from build123d import *

# Parameters (mm, degrees)
SKETCH1_W           = 22.84
SKETCH1_H           = 12.1
BOSS_EXTRUDE1_DEPTH = 17.2
BOSS_EXTRUDE2_DEPTH = 2.48
BOSS_EXTRUDE3_START = 2.48
SKETCH1_4_W         = 22.84
SKETCH1_4_H         = 12.1
BOSS_EXTRUDE3_DEPTH = 4.4
BOSS_EXTRUDE4_START = 6.88
SKETCH1_5_R         = 2.8
SKETCH1_5_R_2       = 6.05
SKETCH1_5_R_3       = 2.35
BOSS_EXTRUDE4_DEPTH = 4.28
BOSS_EXTRUDE5_START = 11.16
SKETCH1_6_R         = 2.35
BOSS_EXTRUDE5_DEPTH = 4.02


with BuildPart() as part:
    # Sketch1 → Boss-Extrude1 (new body)
    with BuildSketch(Plane(origin=(0, 0, 0), x_dir=(1, 0, 0), z_dir=(0, 1, 0))):
        with Locations((5.37, 0)):
            Rectangle(SKETCH1_W, SKETCH1_H)
    extrude(amount=-BOSS_EXTRUDE1_DEPTH)

    # Sketch1<3> → Boss-Extrude2 (add)
    with BuildSketch(Plane(origin=(0, 0, 0), x_dir=(1, 0, 0), z_dir=(0, 1, 0))):
        with BuildLine():
            Line((21.48, -6.05), (21.48, -1))
            Line((21.48, -1), (19.07, -1))
            ThreePointArc((19.07, -1), (18.07, 0), (19.07, 1))
            Line((19.07, 1), (21.48, 1))
            Line((21.48, 1), (21.48, 6.05))
            Line((21.48, 6.05), (-10.74, 6.05))
            Line((-10.74, 6.05), (-10.74, 1.33332999))
            Line((-10.74, 1.33332999), (-8.33, 1.33332999))
            ThreePointArc((-8.33, 1.33332999), (-6.99667001, 0), (-8.33, -1.33332999))
            Line((-8.33, -1.33332999), (-10.74, -1.33332999))
            Line((-10.74, -1.33332999), (-10.74, -6.05))
            Line((-10.74, -6.05), (21.48, -6.05))
        make_face()
    extrude(amount=BOSS_EXTRUDE2_DEPTH)

    # Sketch1<4> → Boss-Extrude3 (add)
    with BuildSketch(Plane(origin=(0, 0, 0), x_dir=(1, 0, 0), z_dir=(0, 1, 0)).offset(BOSS_EXTRUDE3_START)):
        with Locations((5.37, 0)):
            Rectangle(SKETCH1_4_W, SKETCH1_4_H)
    extrude(amount=BOSS_EXTRUDE3_DEPTH)

    # Sketch1<5> → Boss-Extrude4 (add)
    # profile 1 of 9: a face of its own
    with BuildSketch(Plane(origin=(0, 0, 0), x_dir=(1, 0, 0), z_dir=(0, 1, 0)).offset(BOSS_EXTRUDE4_START)):
        with Locations((7, 0)):
            Circle(SKETCH1_5_R)
    # profile 2 of 9: a face of its own
    with BuildSketch(Plane(origin=(0, 0, 0), x_dir=(1, 0, 0), z_dir=(0, 1, 0)).offset(BOSS_EXTRUDE4_START)):
        Circle(SKETCH1_5_R_2)
        Circle(SKETCH1_5_R_3, mode=Mode.SUBTRACT)
    # profile 3 of 9: a face of its own
    with BuildSketch(Plane(origin=(0, 0, 0), x_dir=(1, 0, 0), z_dir=(0, 1, 0)).offset(BOSS_EXTRUDE4_START)):
        with BuildLine():
            Line((4.691578101, -3.819894622), (7.957656401, -2.631139338))
            ThreePointArc((7.957656401, -2.631139338), (6.72964006, -2.786916845), (5.554464286, -2.398004691))
            ThreePointArc((5.554464286, -2.398004691), (5.172116481, -3.138743556), (4.691578101, -3.819894622))
        make_face()
    # profile 4 of 9: a face of its own
    with BuildSketch(Plane(origin=(0, 0, 0), x_dir=(1, 0, 0), z_dir=(0, 1, 0)).offset(BOSS_EXTRUDE4_START)):
        with BuildLine():
            ThreePointArc((5.554464286, 2.398004691), (6.72964006, 2.786916845), (7.957656401, 2.631139338))
            Line((7.957656401, 2.631139338), (4.691578101, 3.819894622))
            ThreePointArc((4.691578101, 3.819894622), (5.172116481, 3.138743556), (5.554464286, 2.398004691))
        make_face()
    # profile 5 of 9: a face of its own
    with BuildSketch(Plane(origin=(0, 0, 0), x_dir=(1, 0, 0), z_dir=(0, 1, 0)).offset(BOSS_EXTRUDE4_START)):
        Circle(SKETCH1_5_R_2)
    # profile 6 of 9: a face of its own
    with BuildSketch(Plane(origin=(0, 0, 0), x_dir=(1, 0, 0), z_dir=(0, 1, 0)).offset(BOSS_EXTRUDE4_START)):
        with Locations((7, 0)):
            Circle(SKETCH1_5_R)
    # profile 7 of 9: a face of its own
    with BuildSketch(Plane(origin=(0, 0, 0), x_dir=(1, 0, 0), z_dir=(0, 1, 0)).offset(BOSS_EXTRUDE4_START)):
        with Locations((7, 0)):
            Circle(SKETCH1_5_R)
    # profile 8 of 9: a face of its own
    with BuildSketch(Plane(origin=(0, 0, 0), x_dir=(1, 0, 0), z_dir=(0, 1, 0)).offset(BOSS_EXTRUDE4_START)):
        Circle(SKETCH1_5_R_2)
    # profile 9 of 9: a face of its own
    with BuildSketch(Plane(origin=(0, 0, 0), x_dir=(1, 0, 0), z_dir=(0, 1, 0)).offset(BOSS_EXTRUDE4_START)):
        Circle(SKETCH1_5_R_3)
    extrude(amount=BOSS_EXTRUDE4_DEPTH)

    # Sketch1<6> → Boss-Extrude5 (add)
    with BuildSketch(Plane(origin=(0, 0, 0), x_dir=(1, 0, 0), z_dir=(0, 1, 0)).offset(BOSS_EXTRUDE5_START)):
        with Locations(Location((0, 0, 0), (0, 0, 270))):
            Circle(SKETCH1_6_R)
    extrude(amount=BOSS_EXTRUDE5_DEPTH)


solid = part.part
Here's how the part is built. I have some questions about the finished solid (model axes, mm). A direction names the side the tool comes from. Round coordinates to 2 decimals unless told otherwise and drop trailing zeros. Loops run counter-clockwise (first coordinate to the right, second up) from the corner with the lowest first, then second, coordinate; pieces in that order, holes last.
1. We'd pull the mould along Z, two halves only. Please class faces 1 (the face through (-7.91, 2.48, -1.43)), 2 (the face through (-6.997, 1.223, -0.029)), 3 (the face through (6.347, 8.99, -3.217)), 4 (the face through (6.302, 8.99, 3.234)): +Z half, -Z half, draft (parallel to the pull), parting line (faces both ways), or undercut.
Answer list:
face 1: draft
face 2: undercut
face 3: -Z half
face 4: +Z half
2. If we section it at B-B on z = 0.5: Write out the boundary of the cut face in (x, y) (3 decimals).
Answer list:
outline: (-7.094, 0) - (-6.05, 0) - (-6.05, -17.2) - (16.79, -17.2) - (16.79, 0) - (18.204, 0) - (18.204, 2.48) - (16.79, 2.48) - (16.79, 6.88) - (9.755, 6.88) - (9.755, 11.16) - (2.296, 11.16) - (2.296, 15.18) - (-2.296, 15.18) - (-2.296, 11.16) - (-6.029, 11.16) - (-6.029, 6.88) - (-6.05, 6.88) - (-6.05, 2.48) - (-7.094, 2.48) - close
3. If I drill on line 1 along Y through (x, z) = (15, -5.25); line 2 along X through (y, z) = (-2, -1.75); line 3 along Y through (x, z) = (4.5, 0), over which ranges is the centre line in solid material (lowest first)?
Answer list:
line 1: y = -17.2 to 6.88
line 2: x = -6.05 to 16.79
line 3: y = -17.2 to 11.16
4. If we section it at A-A on y = -13: Write out the boundary of the cut face in (x, z).
Answer list:
outline: (-6.05, -6.05) - (16.79, -6.05) - (16.79, 6.05) - (-6.05, 6.05) - close
5. For P1, Ø5, axis at x = -3.5, z = 2, coming from the +Y side; P2, Ø3.5, axis at x = 6.5, z = -1.5, coming from the +Y side; P3, Ø2, axis at y = -9.5, z = 4.5, coming from the +X side; P4, Ø3.5, axis at y = -4.5, z = 0.5, coming from the -X side, each with a flat end and sliding along its axis, tell me the tip position at first contact or that it passes through.
Answer list:
P1: stops at y = 15.18
P2: stops at y = 11.16
P3: stops at x = 16.79
P4: stops at x = -6.05
6. Which directions (+Z, -Z, +X, -X, +Y, -Y) give clear straight access to the entire face, cutting with the end or side of a thin tool? Please do faces 5 (the face through (-5, 6.88, -5)), 6 (the face through (19.1, 2.48, -1.4)), 7 (the face through (4, 11.16, 0)), 8 (the face through (19.1, 0, -1.4)), 9 (the face through (-5, 6.88, 5)).
Answer list:
face 5: -Z, -X, +Y
face 6: +Z, -Z, +X, +Y
face 7: +Y
face 8: +Z, -Z, +X, -Y
face 9: +Z, -X, +Y
7. If we section it at C-C on x = 11.5: Write out the boundary of the cut face in (y, z).
Answer list:
outline: (-17.2, -6.05) - (6.88, -6.05) - (6.88, 6.05) - (-17.2, 6.05) - close
8. If we section it at D-D on z = -5.25: Write out the boundary of the cut face in (x, y).
Answer list:
outline: (-10.74, 0) - (-6.05, 0) - (-6.05, -17.2) - (16.79, -17.2) - (16.79, 0) - (21.48, 0) - (21.48, 2.48) - (16.79, 2.48) - (16.79, 6.88) - (3.01, 6.88) - (3.01, 11.16) - (-3.01, 11.16) - (-3.01, 6.88) - (-6.05, 6.88) - (-6.05, 2.48) - (-10.74, 2.48) - close
